CAD build for the part. Positions are in the model's coordinates, mm. A direction names the side the tool comes from. Round coordinates to 2 decimals unless told otherwise and drop trailing zeros. Order: outer loops, then holes, each group sorted by start corner. A loop starts at its lowest first (then second) coordinate and runs counter-clockwise, first axis right, second up. Notation, with made-up numbers: (-27, -18) -> (-12, -18) arc R25 ccw to (-12, 9) -> close; hole circle Ø3 at (-36, -20). An arc over 180 degrees is marked (long way). Return JSON: item names as keys, results as strings. Group by question number.
Q1. Cut at D-D (z = -32.5). Write the cut outline in (x, y).
Q2. Which spindle directions (+Z, -Z, +X, -X, +Y, -Y) get a long thin tool onto all of the face, cutting with end or side? Do faces 1 (the flat face through (10, 15, -4.95)), 2 (the flat face through (15, 45, -30)), 3 (the flat face through (-6, 107, -15)), 4 (the cylindrical face through (21.035, 7.973, -10.515)), 5 (the flat face through (0, 62, -15)). Say none if no direction does.
Q3. Probe line 1 along Z through (x, y) = (26, 15); line 2 along Z through (x, y) = (18, 21.5); line 3 along Y through (x, z) = (26.75, -15) (3 decimals). List the from-to ranges inside material, lowest first.
Q4. Cut at B-B (y = 15.06). Write the cut outline in (x, z) (3 decimals), then the cut area to 4 significant figures.
Q5. Flat gauge pins, fed straight in: pin 1 (4.5 mm diameter, centred on x = 15, z = -37.5, fed in from -Y); pin 2 (22 mm diameter, centred on x = 13.5, y = 23, fed in from -Z); pin 3 (9.5 mm diameter, centred on x = -4.5, z = -7, fed in from -Y). Where does each tip first touch, or does it go through?
Q6. Mould opens along Z. For faces 6 (the flat face through (10, 16, -25.05)), 7 (the flat face through (13, 107, 15)), 8 (the flat face through (18, 0, -27)) say: +Z half, -Z half, draft (parallel to the pull), parting line (faces both ways), or undercut.
Q7. Cut at C-C (x = 27). Write the cut outline in (y, z) (3 decimals).
Q8. Cut at A-A (z = -15). Count the separate pieces of the cut face and the enclosed holes in it, then the cut area to 3 significant figures.
Autodesk Inventor part; units mm, degrees
ref_plane "Work Plane1" through (0, 0, -15) normal (0, 0, 1) x (1, 0, 0)
ref_plane "YZ Plane" through (0, 0, 0) normal (1, 0, 0) x (0, 1, 0)
ref_plane "XZ Plane" through (0, 0, 0) normal (0, 1, 0) x (-1, 0, 0)
sketch "Sketch1" plane through (0, 0, 0) normal (0, 0, 1) x (1, 0, 0)
  line L0 (0, 0) -> (25, 0)
  line L1 (25, 0) -> (25, 40)
  line L2 (25, 40) -> (0, 40)
  line L3 (0, 40) -> (0, 0)
  dimension "d1" = 25
  dimension "d2" = 40
  dimension "d3" = 25
extrude "Extrusion1" add sketch "Sketch1" against normal blind 30
sketch "Sketch2" plane through (25, 0, 0) normal (1, 0, 0) x (0, 0, -1)
  line L0 (0, 0) -> (30, 0)
  circle A0 centre (15, 6.56) radius 2.46
extrude "Extrusion2" cut sketch "Sketch2" against normal blind 30
sketch "Sketch3" plane through (0, 0, 0) normal (-1, 0, 0) x (0, 0, 1)
  line L0 (0, 0) -> (-30, 0)
  line L1 (-25.05, 0) -> (-4.95, 0)
  line L2 (-4.95, 0) -> (-4.95, 33.12)
  line L3 (-4.95, 33.12) -> (-25.05, 33.12)
  line L4 (-25.05, 33.12) -> (-25.05, 0)
  dimension "d11" = 20.1
extrude "Extrusion3" cut sketch "Sketch3" against normal blind 20
sketch "Sketch4" plane through (0, 0, 0) normal (0, -1, 0) x (1, 0, 0)
  line L0 (20, -4.95) -> (20, -25.05)
  line L1 (20, -15) -> (25, -15)
  line L2 (25, 0) -> (25, -30)
  line L3 (20, -8.025) -> (25, -8.025)
  line L4 (25, -8.025) -> (25, -21.975)
  line L5 (25, -21.975) -> (20, -21.975)
  line L6 (20, -21.975) -> (20, -8.025)
  line L7 (20, -8.025) -> (25, -21.975) construction
  line L8 (25, -8.025) -> (20, -21.975) construction
  line L9 (25, -12.54) -> (25, -17.46)
  point P0 (0, 0)
  point P1 (22.5, -15)
  dimension "d14" = 13.95
extrude "Extrusion4" add sketch "Sketch4" along normal blind 15
sketch "Sketch5" plane through (20, 0, 0) normal (-1, 0, 0) x (0, 0, 1)
  circle A0 centre (-15, 6.56) radius 2.46
  circle A1 centre (-15, 6.56) radius 4.7025
  circle A2 centre (-15, 6.56) radius 2.46
  circle A3 centre (-15, 6.56) radius 2.46
  point P0 (0, 0)
  dimension "d17" = 9.405
extrude "Extrusion5" cut sketch "Sketch5" against normal blind 2.1
sketch "Sketch6" plane through (25, 0, 0) normal (1, 0, 0) x (0, 0, -1)
  circle A0 centre (15, 6.56) radius 4.7025
  line L0 (15, 6.56) -> (15, 23.56)
  circle A1 centre (15, 23.56) radius 2.46
  point P0 (0, 0)
  dimension "d20" = 17
  dimension "d21" = 4.92
extrude "Extrusion6" cut sketch "Sketch6" against normal blind 10 contours A1
sketch "Sketch7" plane through (20, 0, 0) normal (-1, 0, 0) x (0, 0, 1)
  circle A0 centre (-15, 23.56) radius 2.46
  circle A1 centre (-15, 23.56) radius 4.7025
  point P0 (0, 0)
  dimension "d24" = 9.405
extrude "Extrusion7" cut sketch "Sketch7" against normal blind 2.1
sketch "Sketch9" plane through (25, 0, 0) normal (1, 0, 0) x (0, 0, -1)
  circle A0 centre (15, 6.56) radius 2.46
  circle A1 centre (15, 6.56) radius 2.46
  circle A2 centre (15, 23.56) radius 2.46
  circle A3 centre (15, 23.56) radius 2.46
  line L0 (30, 40) -> (30, 0)
  line L1 (30, 0) -> (30, 40)
  line L2 (30, 40) -> (0, 40)
  line L3 (0, 40) -> (0, 0)
  line L4 (0, 0) -> (8.025, 0)
  line L5 (21.975, 0) -> (21.975, -15)
  line L6 (21.975, -15) -> (8.025, -15)
  line L7 (8.025, -15) -> (8.025, 0)
  line L8 (0, 0) -> (8.025, 0)
  line L9 (21.975, 0) -> (30, 0)
extrude "Extrusion8" add sketch "Sketch9" along normal blind 5
sketch "Sketch10" plane through (0, 40, 0) normal (0, 1, 0) x (1, 0, 0)
  line L0 (0, 30) -> (30, 30)
  line L1 (30, 0) -> (0, 0)
  line L2 (0, 30) -> (30, 30)
  line L3 (30, 30) -> (30, 0)
  line L4 (30, 0) -> (0, 0)
  line L5 (0, 0) -> (0, 30)
extrude "Extrusion9" add sketch "Sketch10" along normal blind 30
sketch "Sketch12" plane through (30, 0, 0) normal (1, 0, 0) x (0, 0, -1)
  circle A0 centre (15, 6.56) radius 2.46
  line L0 (15, 6.56) -> (15, 15.06)
  circle A1 centre (15, 15.06) radius 2.525
  point P0 (0, 0)
  dimension "d31" = 8.5
  dimension "d33" = 5.05
extrude "Extrusion10" cut sketch "Sketch12" against normal blind 30 contours A1
sketch "Sketch14" plane through (0, 0, 0) normal (0, 0, 1) x (1, 0, 0)
  line L0 (30, 70) -> (0, 70)
  line L1 (0, 70) -> (0, 85)
  line L2 (30, 0) -> (30, 70)
  line L3 (30, 109) -> (30, 70)
  line L4 (30, 105) -> (30, 100)
  line L5 (-12, 124) -> (15, 124)
  line L6 (-8, 122) -> (-12, 124)
  line L7 (-8, 122) -> (-4, 112)
  line L8 (-8, 102) -> (-12, 100)
  line L9 (-8, 102) -> (-4, 112)
  line L10 (30, 109) -> (15, 124)
  line L11 (0, 85) -> (0, 100)
  line L12 (0, 100) -> (-12, 100)
  point P0 (0, 0)
  dimension "d69" = 12
extrude "Extrusion12" add sketch "Sketch14" against normal blind 30
sketch "Sketch15" plane through (0, 0, -25.05) normal (-1, 0, 0) x (0, 0, 1)
  line L0 (0, 33.12) -> (20.1, 33.12)
  line L1 (20.1, 33.12) -> (20.1, 0)
  line L2 (0, 33.12) -> (20.1, 33.12)
  line L3 (20.1, 33.12) -> (20.1, 31.1)
  line L4 (20.1, 31.1) -> (0, 31.1)
  line L5 (0, 31.1) -> (0, 33.12)
  point P0 (25.05, 0)
  dimension "d57" = 2.02
extrude "Extrusion13" add sketch "Sketch15" against normal blind 20
sketch "Sketch19" plane through (0, 0, 0) normal (0, 0, 1) x (1, 0, 0)
  line L0 (0, 100) -> (-12, 100)
  line L1 (0, 100) -> (-12, 100)
  line L2 (-12, 100) -> (-8, 102)
  line L3 (-12, 100) -> (-8, 102)
  line L4 (-8, 102) -> (-4, 112)
  line L5 (-8, 102) -> (-4, 112)
  line L6 (-4, 112) -> (-8, 122)
  line L7 (-4, 112) -> (-8, 122)
  line L8 (-8, 122) -> (-12, 124)
  line L9 (-8, 122) -> (-12, 124)
  line L10 (-12, 124) -> (15, 124)
  line L11 (-12, 124) -> (15, 124)
  line L12 (15, 124) -> (30, 109)
  line L13 (15, 124) -> (30, 109)
  line L14 (30, 109) -> (30, 89)
  line L15 (30, 89) -> (0, 89)
  line L16 (0, 89) -> (0, 100)
  point P0 (0, 0)
  dimension "d71" = 20
  dimension "d72" = 30
extrude "Extrusion14" add sketch "Sketch19" along normal blind 15
ref_plane "Work Plane1" through (0, 0, -15) normal (0, 0, 1) x (1, 0, 0)
mirror "Mirror1" about plane through (0, 0, -15) normal (0, 0, 1) of "Extrusion14"
properties part number "rec_b_20mm_x_60mm"
Solution:
{
 "1": {"outline": "(-12, 100) -> (0, 100) -> (0, 89) -> (30, 89) -> (30, 109) -> (15, 124) -> (-12, 124) -> (-8, 122) -> (-4, 112) -> (-8, 102) -> close"},
 "2": {"face 1": "-X, -Y", "face 2": "-Z, +X, -X, -Y", "face 3": "+Z, -Z, -X", "face 4": "-X", "face 5": "+Z, -Z, -X, -Y"},
 "3": {"line 1": "z = -30 to -17.52, -12.48 to 0", "line 2": "z = -30 to -25.05, -4.95 to 0", "line 3": "y = -15 to 4.1, 9.02 to 12.535, 17.585 to 21.1, 26.02 to 112.25"},
 "4": {"outline": "(0, -30) -> (30, -30) -> (30, -17.525) -> (20, -17.525) -> (20, -25.05) -> (0, -25.05) -> close; (0, -4.95) -> (20, -4.95) -> (20, -12.475) -> (30, -12.475) -> (30, 0) -> (0, 0) -> close", "area": "447.5 mm²"},
 "5": {"pin 1": "stops at y = 89", "pin 2": "stops at z = -30", "pin 3": "stops at y = 31.1"},
 "6": {"face 6": "undercut", "face 7": "+Z half", "face 8": "draft"},
 "7": {"outline": "(-15, -21.975) -> (0, -21.975) -> (0, -30) -> (89, -30) -> (89, -45) -> (112, -45) -> (112, 15) -> (89, 15) -> (89, 0) -> (0, 0) -> (0, -8.025) -> (-15, -8.025) -> close; hole circle Ø4.92 at (6.56, -15); hole circle Ø5.05 at (15.06, -15); hole circle Ø4.92 at (23.56, -15)"},
 "8": {"separate pieces": "4", "enclosed holes": "0", "area": "3,130 mm²"}
}
